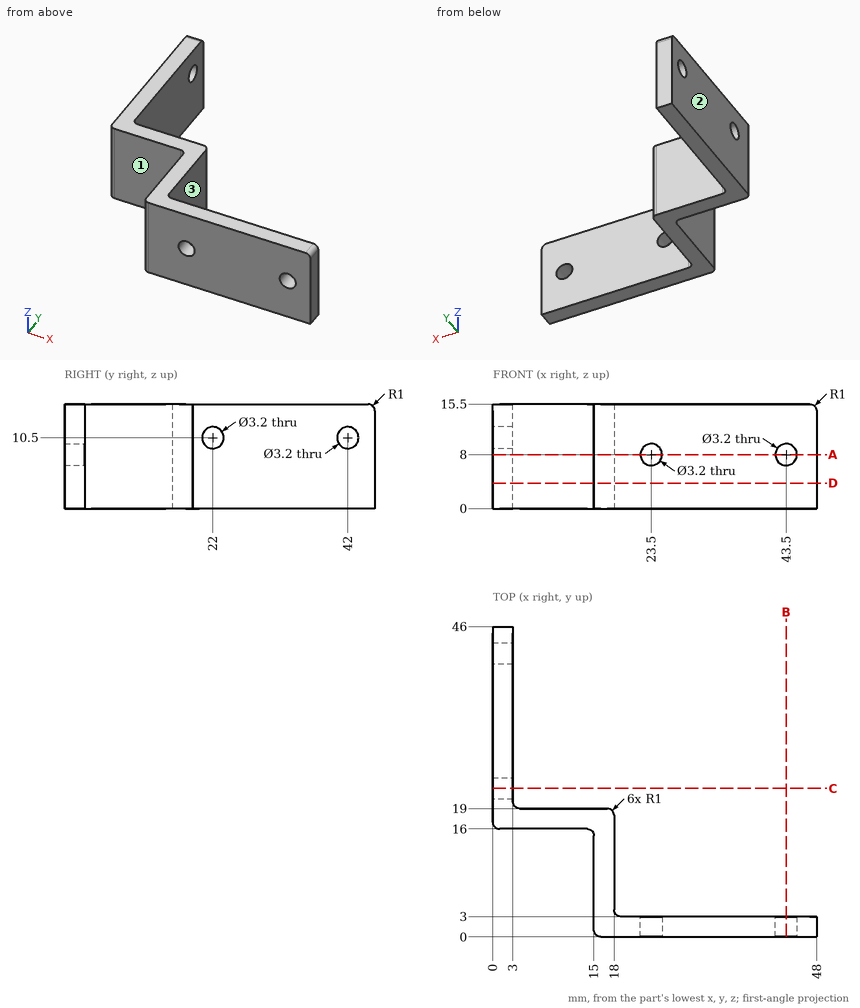
Geometry: see drawing. Coordinates: mm, zero at the bounding-box minimum. A direction names the side the tool comes from. Round coordinates to 2 decimals unless told otherwise and drop trailing zeros. Loops run counter-clockwise (first coordinate to the right, second up) from the corner with the lowest first, then second, coordinate; pieces in that order, holes last. Notation, with made-up numbers: M 87.5,23 L 116.5,23 A27 cw 116.5,60 Z; hole C -14.5,5.25 d10. An arc over 180 degrees is marked long. Use a Markdown table: item, result. Add a question column.
1. Section query C-C on y = 22. Return the cut outline in (x, z), then the cut area to 3 significant figures.
2. Section query A-A on z = 8. Return the cut outline in (x, y), then the cut area to 3 significant figures.
3. Line query: line 1 (Z direction, x = 1.5, y = 42); line 2 (Z direction, x = 23.5, y = 1.1); line 3 (X direction, y = 30, z = 1.5). Output: solid intervals per line, ascending.
4. Section query D-D on z = 3.75. Return the cut outline in (x, y).
5. Section query B-B on x = 43.5. Return the cut outline in (y, z).
6. Reachability of the marked faces 1, 2 and 3 from +Z, -Z, +X, -X, +Y, -Y: full face, straight path, thin tool, end or side. Return the list, or none.
7. Contact query for flat-ended pins moving along their axis: P1, Ø4, axis at x = 30, z = 10, coming from the +Y side; P2, Ø12, axis at x = 11.5, y = 35, coming from the -Z side; P3, Ø2, axis at x = 6.5, z = 6, coming from the -Y side; P4, Ø1.5, axis at y = 19, z = 12, coming from the +X side. Output: stop coordinate, or through.
Reported:
| question | item | result |
|---|---|---|
| 1 | outline | M 0,0 L 3,0 L 3,8.9 L 0,8.9 Z; M 0,12.1 L 3,12.1 L 3,15.5 L 0,15.5 Z |
| 1 | area | 36.9 mm² |
| 2 | outline | M 0,17 A1 ccw 1,16 L 14,16 A1 cw 15,15 L 15,1 A1 ccw 16,0 L 21.9,0 L 21.9,3 L 19,3 A1 cw 18,4 L 18,18 A1 ccw 17,19 L 4,19 A1 cw 3,20 L 3,46 L 0,46 Z; M 25.1,0 L 41.9,0 L 41.9,3 L 25.1,3 Z; M 45.1,0 L 48,0 L 48,3 L 45.1,3 Z |
| 2 | area | 254 mm² |
| 3 | line 1 | z = 0 to 8.9, 12.1 to 15.5 |
| 3 | line 2 | z = 0 to 6.4, 9.6 to 15.5 |
| 3 | line 3 | x = 0 to 3 |
| 4 | outline | M 0,17 A1 ccw 1,16 L 14,16 A1 cw 15,15 L 15,1 A1 ccw 16,0 L 48,0 L 48,3 L 19,3 A1 cw 18,4 L 18,18 A1 ccw 17,19 L 4,19 A1 cw 3,20 L 3,46 L 0,46 Z |
| 5 | outline | M 0,0 L 3,0 L 3,6.4 L 0,6.4 Z; M 0,9.6 L 3,9.6 L 3,15.5 L 0,15.5 Z |
| 6 | face 1 | +Z, -Z, -X, -Y |
| 6 | face 2 | +Z, -Z, -X, +Y, -Y |
| 6 | face 3 | +Z, -Z, +X, +Y |
| 7 | P1 | stops at y = 3 |
| 7 | P2 | passes through |
| 7 | P3 | stops at y = 16 |
| 7 | P4 | stops at x = 17.97 |
